Verification items for this drawing (mm, ordinates from the low corner). A direction names the side the tool comes from. Round coordinates to 2 decimals unless told otherwise and drop trailing zeros. Loops run counter-clockwise (first coordinate to the right, second up) from the corner with the lowest first, then second, coordinate; pieces in that order, holes last. Notation, with made-up numbers: (63.5, 25.25) - (96.5, 25.25) arc R11 cw to (96.5, 42.25) - close; hole circle Ø5 at (28, -21). An arc over 180 degrees is marked (long way). Put each result on its own line as item: value. Start each with the question number.
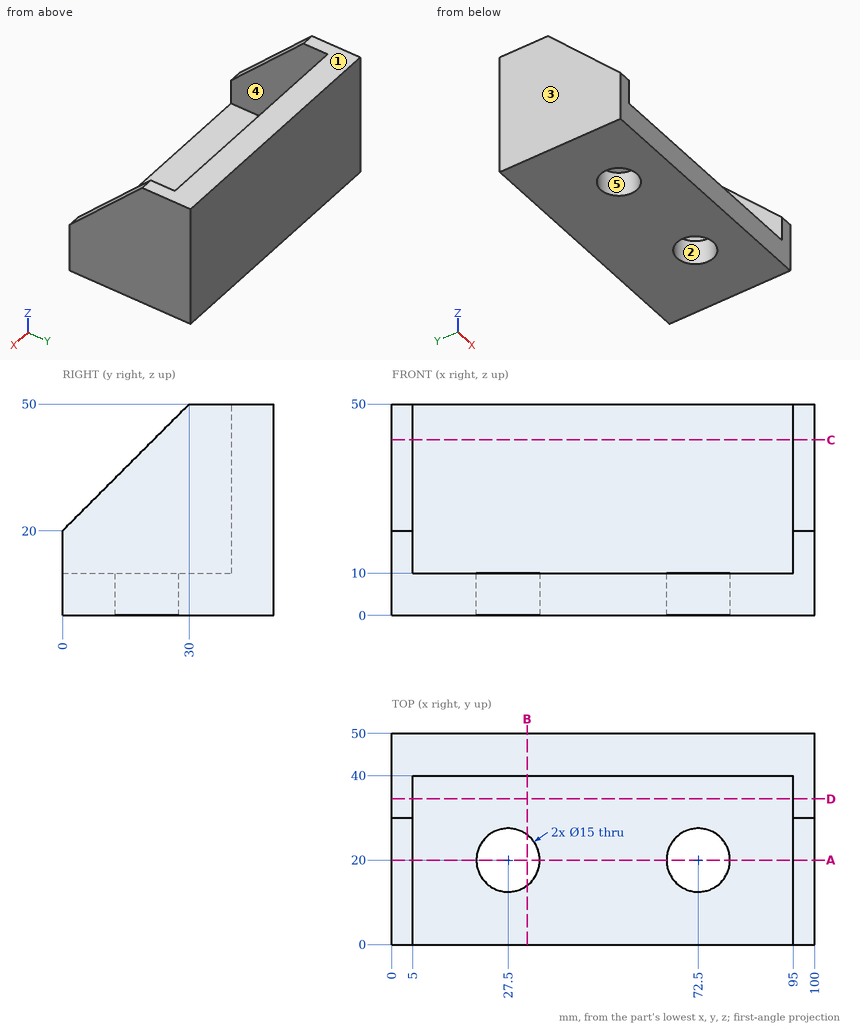
Q1. Cross-section at C-C on z = 41.5. Enter the section's corners in (x, y), and give its area (4 significant figures).
Q2. Cross-section at D-D on y = 34.5. Enter the section's corners in (x, z).
Q3. Depth check by flat-ended pin: pin 1 Ø5 at (x, z) = (53, 19.5) entering from -Y; pin 2 Ø1.5 at (x, y) = (38, 41) entering from -Z; pin 3 Ø1 at (x, y) = (48, 39) entering from +Z. Enter the tip coordinate at first touch or a pass-through.
Q4. Draft check along X on the marked faces 1, 2 and 3. Enter one of: +X half, -X half, draft (parallel to the pull), parting line (faces both ways), or undercut.
Q5. Set-up check for the marked faces 4 and 5: record each of +Z, -Z, +X, -X, +Y, -Y from which the full face is reachable in a straight line by a thin tool's end or side.
Q6. Material ranges on line 1 (X direction, y = 8.5, z = 16); line 2 (X direction, y = 17.5, z = 9); line 3 (Y direction, x = 27.5, z = 6.5), recorded low to high. Write a range as from..to.
Q7. Cross-section at A-A on y = 20. Enter the section's corners in (x, z), and give its area (3 significant figures).
Q8. Cross-section at B-B on x = 32. Enter the section's corners in (y, z), and give its area (3 significant figures).
Answer list:
1. outline: (0, 21.5) - (5, 21.5) - (5, 40) - (95, 40) - (95, 21.5) - (100, 21.5) - (100, 50) - (0, 50) - close
1. area: 1,185 mm2
2. outline: (0, 0) - (100, 0) - (100, 50) - (95, 50) - (95, 10) - (5, 10) - (5, 50) - (0, 50) - close
3. pin 1: stops at y = 40
3. pin 2: stops at z = 0
3. pin 3: stops at z = 10
4. face 1: draft
4. face 2: undercut
4. face 3: -X half
5. face 4: +Z, -Y
5. face 5: +Z, -Z
6. line 1: x = 0..5, 95..100
6. line 2: x = 0..20.43, 34.57..65.43, 79.57..100
6. line 3: y = 0..12.5, 27.5..50
7. outline: (0, 0) - (20, 0) - (20, 10) - (5, 10) - (5, 40) - (0, 40) - close; (35, 0) - (65, 0) - (65, 10) - (35, 10) - close; (80, 0) - (100, 0) - (100, 40) - (95, 40) - (95, 10) - (80, 10) - close
7. area: 1,000 mm2
8. outline: (0, 0) - (14, 0) - (14, 10) - (0, 10) - close; (26, 0) - (50, 0) - (50, 50) - (40, 50) - (40, 10) - (26, 10) - close
8. area: 780 mm2
